Verification items for this drawing (mm, ordinates from the low corner). Give positions to 0.01 mm unless a question says otherwise; leave off trailing zeros. Loops run counter-clockwise (first coordinate to the right, second up) from the corner with the lowest first, then second, coordinate; pieces in that order, holes last. Notation, with made-up numbers: M 41,42.25 L 67,42.25 A8 ccw 67,46.25 Z; hole C -0.75,31 d8. An arc over 180 degrees is marked long. Answer in a Markdown table with one row per item.
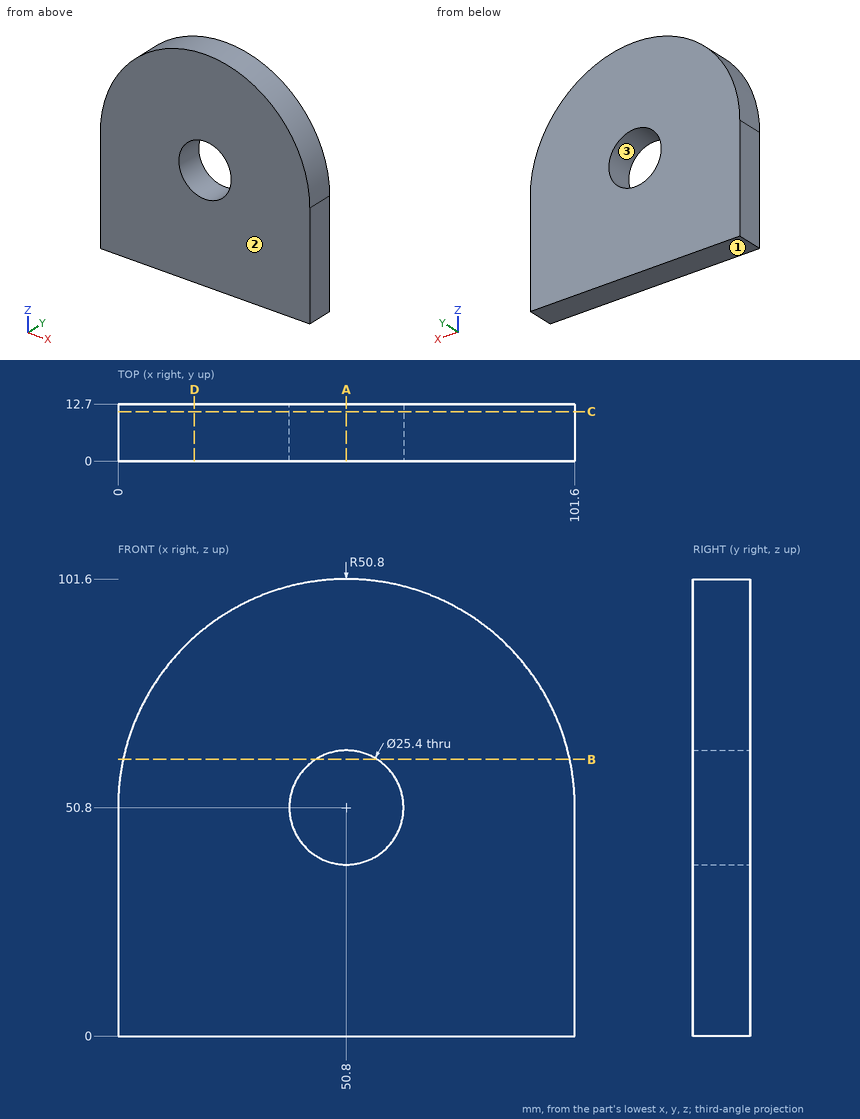
Item 1: Sectioned sample at A-A (x = 50.8). Record the cut outline in (y, z), and give its area (3 significant figures).
Reported:
| item | result |
|---|---|
| outline | M 0,0 L 12.7,0 L 12.7,38.1 L 0,38.1 Z; M 0,63.5 L 12.7,63.5 L 12.7,101.6 L 0,101.6 Z |
| area | 968 mm^2 |
Item 2: Sectioned sample at C-C (y = 11). Record the cut outline in (x, z), and give its area (3 significant figures).
Reported:
| item | result |
|---|---|
| outline | M 0,0 L 101.6,0 L 101.6,50.8 A50.8 ccw 0,50.8 Z; hole C 50.8,50.8 d25.4 |
| area | 8,710 mm^2 |
Item 3: Sectioned sample at D-D (x = 17). Record the cut outline in (y, z), and give its area (3 significant figures).
Reported:
| item | result |
|---|---|
| outline | M 0,0 L 12.7,0 L 12.7,88.72 L 0,88.72 Z |
| area | 1,130 mm^2 |
Item 4: Sectioned sample at B-B (z = 61.5). Record the cut outline in (x, y).
Reported:
| item | result |
|---|---|
| outline | M 1.14,0 L 43.96,0 L 43.96,12.7 L 1.14,12.7 Z; M 57.64,0 L 100.46,0 L 100.46,12.7 L 57.64,12.7 Z |
Item 5: Scan lines: L1, parallel to Z at x = 50.8, y = 8.5; L2, parallel to X at y = 5.25, z = 59.5; L3, parallel to Z at x = 48, y = 9. Record each from-to range of solid material in increasing order. Write a range as [from, to].
Reported:
| item | result |
|---|---|
| L1 | z = [0, 38.1], [63.5, 101.6] |
| L2 | x = [0.75, 41.55], [60.05, 100.85] |
| L3 | z = [0, 38.41], [63.19, 101.52] |
Item 6: Go/stop test with flat-tipped pins: pin 1 (3 mm diameter, centred on x = 61, y = 11, fed in from +Z); pin 2 (1.5 mm diameter, centred on x = 50.5, y = 4, fed in from +Z). Record where each tip stops, or that it passes through.
Reported:
| item | result |
|---|---|
| pin 1 | stops at z = 100.85 |
| pin 2 | stops at z = 101.6 |
Item 7: Release check for a two-part mould opening along Z. For the marked faces 1, 2 and 3 record: released by +Z, released by -Z, zero draft, split by the parting line, or undercut.
Reported:
| item | result |
|---|---|
| face 1 | released by -Z |
| face 2 | zero draft |
| face 3 | undercut |
